Geometry: final body of the model. Coordinates: model frame, mm. Give positions to 0.01 mm unless a question says otherwise; leave off trailing zeros. Write each loop counter-clockwise with the first axis right and the second up, starting at its lowest first coordinate (ties: lowest second). Pieces come first, ordered by that corner, then holes. Notation, with made-up numbers: (67.5, -5) -> (86.5, -5) arc R12 cw to (86.5, 14) -> close; hole circle Ø6 at (72.25, 13.5). An arc over 180 degrees is marked (long way). Answer as a JSON object with one key per item and string values. Group by question number.
(1) Section query D-D on x = -9. Output: boundary loops of the cut face in (y, z) (3 decimals), plus the area to 3 significant figures.
(2) Section query C-C on z = 2. Output: boundary loops of the cut face in (x, y), plus the area to 3 significant figures.
(3) Section query B-B on y = 0. Output: boundary loops of the cut face in (x, z).
(4) Material intervals for probe 1 along Y at (x, z) = (-18, -1.5); probe 2 along Y at (x, z) = (-11, 4.5) (3 decimals); probe 3 along X at (y, z) = (-28.5, 4.25), sorted ascending.
(5) Contact query for flat-ended pins moving along their axis: pin 1 Ø1 at (x, z) = (-12, -3.5) entering from +Y; pin 2 Ø6 at (x, y) = (-45.5, 12.5) entering from +Z; pin 3 Ø1.5 at (x, z) = (-27.5, -2.5) entering from +Y. Output: stop coordinate, or through.
(6) Section query A-A on x = -34. Output: boundary loops of the cut face in (y, z), plus the area to 3 significant figures.
from build123d import *

# Parameters (mm, degrees)
BOSS_EXTRUDE1_DEPTH = 7.5


with BuildPart() as part:
    # Sketch1 → Boss-Extrude1 (new body, symmetric)
    with BuildSketch(Plane.XY):
        with BuildLine():
            Line((-70, 75), (-40, 75))
            Line((-40, 75), (0, 50))
            ThreePointArc((0, 50), (-50, 0), (0, -50))
            Line((0, -50), (-40, -75))
            Line((-40, -75), (-70, -75))
            Line((-70, -75), (-70, 75))
        make_face()
    extrude(amount=BOSS_EXTRUDE1_DEPTH, both=True)


solid = part.part
Answer list:
{
 "1": {"outline": "(-55.625, -7.5) -> (-49.183, -7.5) -> (-49.183, 7.5) -> (-55.625, 7.5) -> close; (49.183, -7.5) -> (55.625, -7.5) -> (55.625, 7.5) -> (49.183, 7.5) -> close", "area": "193 mm2"},
 "2": {"outline": "(-70, -75) -> (-40, -75) -> (0, -50) arc R50 cw to (0, 50) -> (-40, 75) -> (-70, 75) -> close", "area": "5,570 mm2"},
 "3": {"outline": "(-70, -7.5) -> (-50, -7.5) -> (-50, 7.5) -> (-70, 7.5) -> close"},
 "4": {"probe 1": "-61.25 to -46.65, 46.65 to 61.25", "probe 2": "-56.875 to -48.775, 48.775 to 56.875", "probe 3": "-70 to -41.08"},
 "5": {"pin 1": "y = 57.81", "pin 2": "z = 7.5", "pin 3": "y = 67.66"},
 "6": {"outline": "(-71.25, -7.5) -> (-36.66, -7.5) -> (-36.66, 7.5) -> (-71.25, 7.5) -> close; (36.66, -7.5) -> (71.25, -7.5) -> (71.25, 7.5) -> (36.66, 7.5) -> close", "area": "1,040 mm2"}
}
